Design review of the part built by this model. Coordinates are the model's own, in mm. A direction names the side the tool comes from. Coordinates: 2 decimals unless noted, no trailing zeros. Write each loop counter-clockwise with the first axis right and the second up, starting at its lowest first coordinate (ties: lowest second). Pieces come first, ordered by that corner, then holes. Notation, with made-up numbers: (63.5, 23) - (106.5, 23) arc R17 ccw to (106.5, 29) - close; hole circle Ø2 at (-28, 45.5). An arc over 180 degrees is marked (long way). One line per item, written item: value.
from build123d import *

# Parameters (mm, degrees)
SKETCH_1_W                                 = 144
SKETCH_1_H                                 = 184
EXTRUDE_1_DEPTH                            = 50
SKETCH_2_R                                 = 3.45
EXTRUDE_2_DEPTH                            = 43.56
MIRROR_1_AT_THE_SECOND_PLANE_COPY_1_SKET_R = 3.45
MIRROR_1_AT_THE_SECOND_PLANE_COPY_1_DEPTH  = 43.56


with BuildPart() as part:
    # Sketch 1 → Extrude 1 (new body)
    with BuildSketch(Plane(origin=(0, 0, 0), x_dir=(1, 0, 0), z_dir=(0, 1, 0))):
        with Locations((-0.153518124, -55.002132196)):
            Rectangle(SKETCH_1_W, SKETCH_1_H)
    extrude(amount=EXTRUDE_1_DEPTH)

    # Sketch 2 → Extrude 2 (add)
    with BuildSketch(Plane.ZY.offset(72.153518124)):
        with Locations(Location((-14.997867804, 19, 0), (0, 0, 180))):
            Circle(SKETCH_2_R)
    extrude_2 = extrude(amount=EXTRUDE_2_DEPTH)

    # Mirror 1: Extrude 2 across plane
    add(extrude_2.mirror(Plane.ZY.offset(0.153518124)))

    # Mirror 1 at the second plane: Extrude 2 across plane
    add(extrude_2.mirror(Plane(origin=(0, 0, 55.002132196), x_dir=(1, 0, 0), z_dir=(0, 0, -1))))

    # Mirror 1 at the second plane copy 1 sket → Mirror 1 at the second plane copy 1 (add)
    with BuildSketch(Plane(origin=(71.846481876, 0, 110.004264392), x_dir=(0, 0, -1), z_dir=(1, 0, 0))):
        with Locations(Location((-14.997867804, 19, 0), (0, 0, 180))):
            Circle(MIRROR_1_AT_THE_SECOND_PLANE_COPY_1_SKET_R)
    extrude(amount=MIRROR_1_AT_THE_SECOND_PLANE_COPY_1_DEPTH)


solid = part.part
1. Consider section D-D, the plane y = 3. Write out the cut boundary in (x, z), then the cut area to 3 significant figures.
Answer block:
outline: (-72.15, -37) - (71.85, -37) - (71.85, 147) - (-72.15, 147) - close
area: 26,500 mm^2
2. Consider section C-C, the plane z = 93.5. Write out the cut boundary in (x, y), then the cut area to 3 significant figures.
Answer block:
outline: (-72.15, 0) - (71.85, 0) - (71.85, 50) - (-72.15, 50) - close
area: 7,200 mm^2
3. Consider section B-B, the plane x = -80.5. Write out the cut boundary in (y, z), then the cut area to 3 significant figures.
Answer block:
outline: circle Ø6.9 at (19, -15); circle Ø6.9 at (19, 125)
area: 74.8 mm^2
4. Mouldability with a two-part tool opening along Z and no side actions: class faces 4 (the face through (93.32, 16.09, -16.85)), 5 (the face through (-1, 25, -36.998)), 6 (the face through (-1, 50, 54)) as released by +Z, released by -Z, zero draft, split by the parting line, or undercut.
Answer block:
face 4: undercut
face 5: released by -Z
face 6: zero draft
5. Consider section A-A, the plane y = 19. Write out the cut boundary in (x, z).
Answer block:
outline: (-115.71, -18.45) - (-72.15, -18.45) - (-72.15, -37) - (71.85, -37) - (71.85, -18.45) - (115.41, -18.45) - (115.41, -11.55) - (71.85, -11.55) - (71.85, 121.55) - (115.41, 121.55) - (115.41, 128.45) - (71.85, 128.45) - (71.85, 147) - (-72.15, 147) - (-72.15, 128.45) - (-115.71, 128.45) - (-115.71, 121.55) - (-72.15, 121.55) - (-72.15, -11.55) - (-115.71, -11.55) - close
6. Insertion check: pin 1 Ø6 at (y, z) = (13, 17.5) entering from +X; pin 2 Ø10 at (x, z) = (66.5, 8.5) entering from -Y; pin 3 Ø6 at (y, z) = (31.5, 46) entering from -X. Each pin has a flat end and moves straight along its axis. Give the tip position at first contact, or say it passes through.
Answer block:
pin 1: stops at x = 71.85
pin 2: stops at y = 0
pin 3: stops at x = -72.15
7. For faces 1 (the face through (-93.63, 17.96, 128.29)), 2 (the face through (93.32, 17.96, 128.29)), 3 (the face through (-1, 0, 54)), list the 3-axis set-ups (+Z, -Z, +X, -X, +Y, -Y) from which the entire face can be reached by the end or side of a thin tool; tool diameter is ignored.
Answer block:
face 1: -X
face 2: +X
face 3: +Z, -Z, +X, -X, -Y
8. Wall thickness on line 1 along X through (y, z) = (7, 5); line 2 along Z through (x, y) = (-73, 16): over which ranges is each line inside the solid? List them lowest first.
Answer block:
line 1: x = -72.15 to 71.85
line 2: z = -16.7 to -13.29, 123.3 to 126.71
